Check sheet for the modelled part. Datum: model origin and axes. Units: mm. A direction names the side the tool comes from. Coordinates: 2 decimals unless noted, no trailing zeros. Order: outer loops, then holes, each group sorted by start corner. A loop starts at its lowest first (then second) coordinate and runs counter-clockwise, first axis right, second up.
1. Cross-section at B-B (x = -8.5). Enter the section's corners in (y, z), then the cut area to 3 significant figures.
2. Thickness scan on line 1 (X direction, y = 73.5, z = 202.5); line 2 (X direction, y = 83, z = 197.5); line 3 (Z direction, x = -1.5, y = 84). Record the ranges inside material, lowest first.
3. Gauge pin test, flat ends, axial feed: pin 1 Ø3 at (x, y) = (0, 90) entering from -Z; pin 2 Ø5 at (y, z) = (89.5, 195) entering from -X; pin 3 Ø6 at (y, z) = (84.5, 197) entering from +X. Record the tip position at first contact, or that the pin passes through.
4. Cross-section at C-C (z = 201.75). Count the separate pieces of the cut face and the enclosed holes in it, then the cut area to 3 significant figures.
5. Draft check along Y on faces 1 (the flat face through (-0.13, 67.71, 203.58)), 2 (the cylindrical face through (11.84, 75.33, 200.8)), 3 (the flat face through (5.997, 86, 197)). Enter one of: released by +Y, released by -Y, zero draft, split by the parting line, or undercut.
6. Set-up check for faces 4 (the cylindrical face through (-0.33, 95.88, 193.32)), 5 (the flat face through (-7.822, 78.987, 199.471)), 6 (the flat face through (7.625, 78.987, 199.471)): record each of +Z, -Z, +X, -X, +Y, -Y from which the full face is reachable in a straight line by a thin tool's end or side.
7. Cross-section at D-D (y = 87). Enter the section's corners in (x, z), then the cut area to 3 significant figures.
8. Cross-section at A-A (x = 12). Enter the section's corners in (y, z).
```python
from build123d import *

# Parameters (mm, degrees)
SKETCH001_AS_DRAWN_R                   = 2.5
EXTRUDE_DEPTH                          = 3
EXTRUDE_ONTO_SKETCH001_PLACEMENT_ANGLE = 20


with BuildPart() as part:
    # Sketch001 as drawn → Extrude (new)
    with BuildSketch(Plane.XY):
        with BuildLine():
            ThreePointArc((5.996666, 20.3), (0, 26.5), (-5.996666, 20.3))
            Line((-5.996666, 20.3), (-5.996666, 17))
            Line((-5.996666, 17), (-5.996666, 6))
            Line((-5.996666, 6), (-9.7, 6))
            ThreePointArc((-9.7, 6), (-15.5, -0.2), (-9.3, -6))
            Line((-9.3, -6), (-6, -6))
            Line((-6, -6), (6, -6))
            Line((6, -6), (9.3, -6))
            ThreePointArc((9.3, -6), (15.503332, 0), (9.3, 6))
            Line((5.996666, 6), (9.3, 6))
            Line((5.996666, 17), (5.996666, 6))
            Line((5.996666, 20.3), (5.996666, 17))
        make_face()
        with Locations((0, 21.5)):
            Circle(SKETCH001_AS_DRAWN_R, mode=Mode.SUBTRACT)
        with Locations((-10.5, 0)):
            Circle(SKETCH001_AS_DRAWN_R, mode=Mode.SUBTRACT)
        with Locations((10.5, 0)):
            Circle(SKETCH001_AS_DRAWN_R, mode=Mode.SUBTRACT)
    extrude(amount=EXTRUDE_DEPTH)


with BuildPart() as part_1:
    # Extrude onto Sketch001 placement: moved
    add(part.part.moved(Location((0, 72.842742, 200.133789))).rotate(Axis((0, 72.842742, 200.133789), (-1, 0, 0)), EXTRUDE_ONTO_SKETCH001_PLACEMENT_ANGLE))


solid = part_1.part
```
Data:
1. outline: (67.2, 202.19) - (71.43, 200.65) - (72.46, 203.47) - (68.23, 205) - close; (74.25, 199.62) - (78.48, 198.08) - (79.51, 200.9) - (75.28, 202.44) - close
1. area: 27.0 mm2
2. line 1: x = -15.5 to -12.99, -8.01 to 8.01, 12.99 to 15.5
2. line 2: x = -6 to 6
2. line 3: z = 196.07 to 199.27
3. pin 1: stops at z = 193.54
3. pin 2: stops at x = -6
3. pin 3: stops at x = 6
4. separate pieces: 1
4. enclosed holes: 2
4. area: 220 mm2
5. face 1: released by -Y
5. face 2: undercut
5. face 3: zero draft
6. face 4: none
6. face 5: -Z, -X, +Y
6. face 6: -Z, +X, +Y
7. outline: (-6, 194.98) - (6, 194.98) - (6, 198.17) - (-6, 198.17) - close
7. area: 38.3 mm2
8. outline: (67.71, 202) - (70.96, 200.82) - (71.99, 203.64) - (68.74, 204.82) - close; (74.72, 199.45) - (77.97, 198.27) - (79, 201.09) - (75.75, 202.27) - close
